Autodesk Inventor part; units mm, degrees
ref_plane "YZ Plane" through (0, 0, 0) normal (1, 0, 0) x (0, 1, 0)
ref_plane "XZ Plane" through (0, 0, 0) normal (0, 1, 0) x (-1, 0, 0)
ref_plane "XY Plane" through (0, 0, 0) normal (0, 0, 1) x (1, 0, 0)
sketch "Sketch1" plane through (0, 0, 0) normal (0, 0, 1) x (1, 0, 0)
  line L0 (0, 0) -> (9.8884, 0)
  line L1 (9.8884, 5) -> (0, 5)
  line L2 (0, 5) -> (0, 0)
  circle A0 centre (12.3379, 2.5) radius 2.5
  line L3 (14.7874, 5) -> (19.5284, 5)
  arc A1 (14.7874, 5) -> (9.8884, 5) centre (12.3379, 2.5) ccw
  arc A2 (9.8884, 0) -> (14.7874, 0) centre (12.3379, 2.5) ccw
  line L4 (19.5284, 5) -> (55.7874, 5)
  line L5 (14.7874, 0) -> (50.7874, 0)
  line L6 (50.7874, 0) -> (50.7874, -15)
  line L7 (50.7874, -15) -> (55.7874, -15)
  line L8 (55.7874, -15) -> (55.7874, 5)
  dimension "d6" = 5
  dimension "d7" = 3.5
  dimension "d8" = 36
  dimension "d9" = 15
  dimension "d10" = 5
extrude "Extrusion1" add sketch "Sketch1" along normal blind 10
sketch "Sketch2" plane through (14.7874, 5, 0) normal (0, 1, 0) x (1, 0, 0)
  circle A0 centre (13.0191, -5) radius 10
  point P0 (-14.7874, 0)
  dimension "d16" = 20
extrude "Extrusion2" add sketch "Sketch2" along normal blind 3
fillet "Fillet1" radius 2 1 edges at (17.8065, 5, 5)
fillet "Fillet2" radius 2 1 edges at (37.4658, 5, 2.4118)
fillet "Fillet3" radius 2 1 edges at (55.7874, 5, 5)
sketch "Sketch3" plane through (50.7874, -15, 0) normal (-1, 0, 0) x (0, 0, 1)
  circle A0 centre (4.8232, 6.283) radius 6.592
  line L0 (0, 0) -> (10, 0)
  point P0 (0, 15)
extrude "Extrusion3" cut sketch "Sketch3" against normal blind 3
fillet "Fillet4" radius 2 1 edges at (14.7874, 5, 5)
fillet "Fillet5" radius 2 1 edges at (9.8884, 5, 5)
fillet "Fillet6" radius 2 1 edges at (14.7874, 0, 5)
fillet "Fillet7" radius 2 1 edges at (9.8884, 0, 5)
sketch "Sketch4" plane through (0, 0, 0) normal (-1, 0, 0) x (0, 0, 1)
  point P0 (0, 0)
  point P1 (5.1471, 2.6969)
hole "Hole1" at (0, 2.6969, 5.1471) direction (1, 0, 0) diameter 2 depth 2 tip angle 118
properties part number "Rocker1"
Read the model definition and answer for the solid it produces. Units are mm, in the model's axes. A direction names the side the tool comes from. Round coordinates to 2 decimals unless told otherwise and drop trailing zeros. Loops run counter-clockwise (first coordinate to the right, second up) from the corner with the lowest first, then second, coordinate; pieces in that order, holes last. Notation, with made-up numbers: (-32.5, -5.75) -> (25.5, -5.75) arc R19 ccw to (25.5, 21.25) -> close; hole circle Ø6 at (-7, -39.5). An arc over 180 degrees is marked (long way). One line per item, written item: value.
1) A cutting plane is placed at B-B (y = -5.75). Determine the outline of the cut face in (x, z).
Answer list:
outline: (53.79, 0) -> (55.79, 0) -> (55.79, 10) -> (53.79, 10) -> close
2) A cutting plane is placed at C-C (x = 32). Determine the outline of the cut face in (y, z), and give its area (3 significant figures).
Answer list:
outline: (0, 0) -> (5, 0) -> (5, -4.08) -> (8, -4.08) -> (8, 14.08) -> (5, 14.08) -> (5, 10) -> (0, 10) -> close
area: 104 mm²
3) Consider L1, parallel to Y at x = 30, z = 14.25; L2, parallel to Y at x = 21.5, z = 9; L3, parallel to X at y = 0.5, z = 5.5. Determine where each line is inside the solid, lowest interval first. Write a range as [from, to].
Answer list:
L1: y = [5, 8]
L2: y = [0, 8]
L3: x = [0, 10.84], [13.84, 55.79]
4) For faces 4 (the face through (1.014, 3.673, 4.93)), 5 (the face through (50.787, -1, 5)), 6 (the face through (5, 5, 5)), determine the directions among +Z, -Z, +X, -X, +Y, -Y from which every point of the face is accessible in a straight line to the end or side of a thin tool.
Answer list:
face 4: -X
face 5: +Z, -Z, -Y
face 6: +Z, -Z, -X, +Y
5) Flat-ended cylindrical pins translate along their axes: P1, Ø1.5, axis at x = 29, z = 11.5, coming from the -Y side; P2, Ø10, axis at x = 13.5, z = -1, coming from the +Y side; P3, Ø2.5, axis at y = -3, z = 4, coming from the -X side. Find the tip coordinate at first contact, or state that the pin passes through.
Answer list:
P1: stops at y = 5
P2: stops at y = 6
P3: stops at x = 50.79
6) A cutting plane is placed at A-A (y = 4.25). Determine the outline of the cut face in (x, z).
Answer list:
outline: (0, 0) -> (10.55, 0) -> (10.55, 10) -> (0, 10) -> close; (14.12, 0) -> (55.35, 0) -> (55.35, 10) -> (14.12, 10) -> close
7) The mould has two halves that part along Y. Classify faces 1 (the face through (28, 5, -2)), 2 (the face through (9.84, 2.39, 4.93)), 3 (the face through (9.8, 5.1, 5.1)): pulls with the +Y half, pulls with the -Y half, needs draft (parallel to the pull), parting line crosses it, or undercut.
Answer list:
face 1: pulls with the -Y half
face 2: undercut
face 3: pulls with the +Y half
